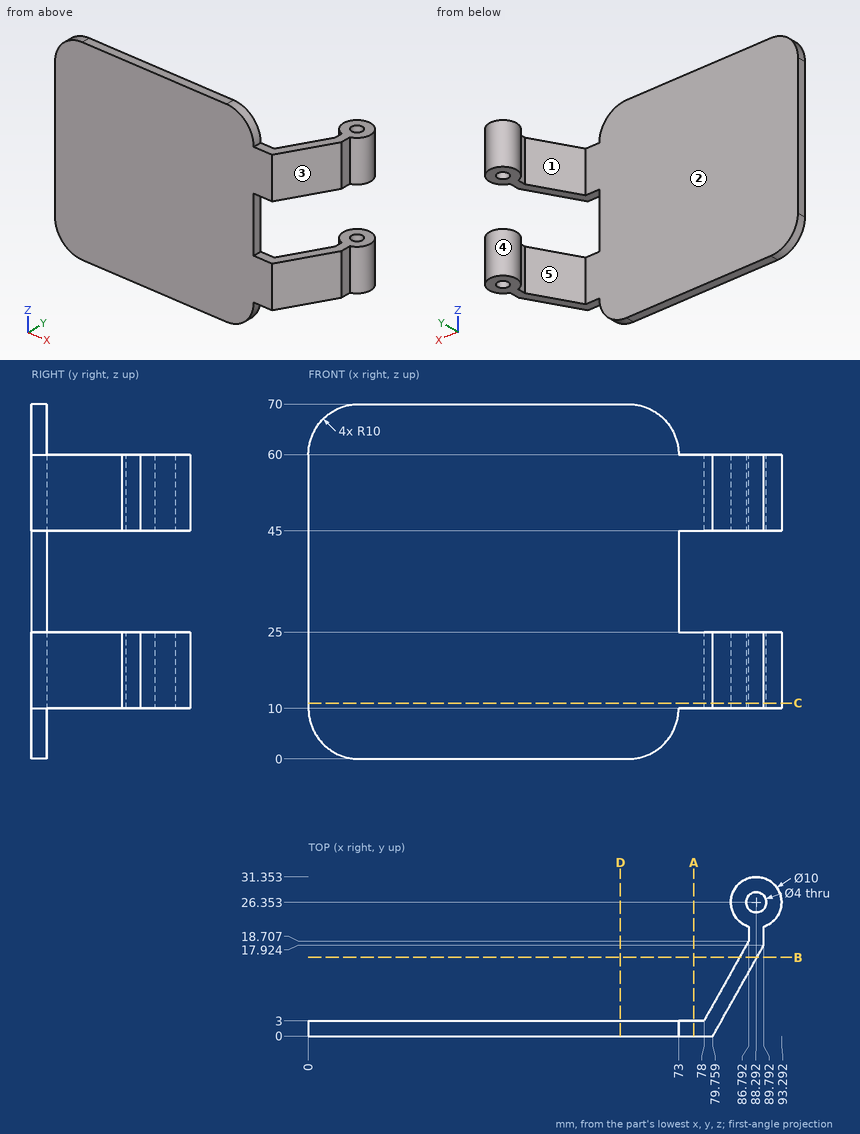
Job drawing, mm, ordinate dimensions from the low corner. One solid piece. A direction names the side the tool comes from. Give positions to 0.01 mm unless a question says otherwise; leave off trailing zeros. Write each loop counter-clockwise with the first axis right and the second up, starting at its lowest first coordinate (ties: lowest second). Pieces come first, ordered by that corner, then holes. Notation, with made-up numbers: (61, -17) -> (95, -17) arc R15 cw to (95, -1) -> close; hole circle Ø7 at (-11, -36.75). An arc over 180 degrees is marked (long way). Return JSON: item names as keys, results as strings.
Item 1: Two-plate mould, pull along Y, no slides. Class the marked faces 1, 2 and 3: +Y half, -Y half, draft (parallel to the pull), parting line (faces both ways), or undercut.
Answer below:
{"face 1": "undercut", "face 2": "+Y half", "face 3": "-Y half"}
Item 2: Band-saw the part on B-B (y = 15.5). List the corners of the cut face in (x, z) (1 decimal), then the cut area to 3 significant figures.
Answer below:
{"outline": "(85, 10) -> (88.4, 10) -> (88.4, 25) -> (85, 25) -> close; (85, 45) -> (88.4, 45) -> (88.4, 60) -> (85, 60) -> close", "area": "103 mm2"}
Item 3: Drop flat-ended pins along their axis: pin 1 (5 mm diameter, centred on x = 88.29, y = 26.35, fed in from +Z); pin 2 (0.9 mm diameter, centred on y = 1, z = 38.5, fed in from +X); pin 3 (3 mm diameter, centred on y = 20.5, z = 19.5, fed in from +X); pin 4 (8 mm diameter, centred on y = 25.5, z = 29.5, fed in from -X). Give the stop position or say it passes through.
Answer below:
{"pin 1": "stops at z = 60", "pin 2": "stops at x = 73", "pin 3": "stops at x = 90.75", "pin 4": "passes through"}
Item 4: Band-saw the part on C-C (z = 11). List the corners of the cut face in (x, y) (1 decimal), then the cut area to 3 significant figures.
Answer below:
{"outline": "(0, 0) -> (79.8, 0) -> (89.8, 17.9) -> (89.8, 21.6) arc R5 ccw (long way) to (86.8, 21.6) -> (86.8, 18.7) -> (78, 3) -> (0, 3) -> close; hole circle Ø4 at (88.3, 26.4)", "area": "370 mm2"}
Item 5: Drill centre lines: probe 1 along Y at (x, z) = (58, 18); probe 2 along X at (y, z) = (19.5, 59); probe 3 along X at (y, z) = (4.5, 16.5). Where is each one in solid material? Low to high.
Answer below:
{"probe 1": "y = 0 to 3", "probe 2": "x = 86.79 to 89.79", "probe 3": "x = 78.84 to 82.28"}
Item 6: Band-saw the part on A-A (x = 76). List the corners of the cut face in (y, z).
Answer below:
{"outline": "(0, 10) -> (3, 10) -> (3, 25) -> (0, 25) -> close; (0, 45) -> (3, 45) -> (3, 60) -> (0, 60) -> close"}
Item 7: Band-saw the part on D-D (x = 61.5). List the corners of the cut face in (y, z), then the cut area to 3 significant figures.
Answer below:
{"outline": "(0, 0) -> (3, 0) -> (3, 70) -> (0, 70) -> close", "area": "210 mm2"}
Item 8: Tool access for the marked faces 4 and 5: list every direction of +Z, -Z, +X, -X, +Y, -Y with a clear straight run to the whole face (end or side of a thin tool).
Answer below:
{"face 4": "+Z, -Z", "face 5": "+Z, -Z, -X"}
